Geometry check sheet. Reference: the model listing, model coordinates, mm. A direction names the side the tool comes from. Round coordinates to 2 decimals unless told otherwise and drop trailing zeros. Order: outer loops, then holes, each group sorted by start corner. A loop starts at its lowest first (then second) coordinate and runs counter-clockwise, first axis right, second up. Notation, with made-up numbers: (11.25, 31.25) -> (52.25, 31.25) arc R25 cw to (52.25, 52.25) -> close; hole circle Ø2 at (15, 60). An arc over 180 degrees is marked (long way). Use a Markdown table: item, result. Add a question column.
Item 1: Sectioned sample at B-B, the plane y = 22. Record the cut outline in (x, z).
Item 2: Sectioned sample at A-A, the plane x = 53. Record the cut outline in (y, z).
Item 3: Sectioned sample at C-C, the plane z = -48.5. Record the cut outline in (x, y).
Item 4: Material ranges on probe 1 along Z at (x, y) = (94, 0.8); probe 2 along Z at (x, y) = (68, 0.95); probe 3 along X at (y, z) = (0.85, 83), recorded low to high. Write a range as [from, to].
Item 5: Set-up check for faces 1 (the flat face through (63, 19, 74.035)), 2 (the flat face through (1, 0, 1)): record each of +Z, -Z, +X, -X, +Y, -Y from which the full face is reachable in a straight line by a thin tool's end or side.
Item 6: Gauge pin test, flat ends, axial feed: pin 1 Ø1.6 at (x, z) = (-94, -19.8) entering from -Y; pin 2 Ø2.5 at (x, z) = (98, -10) entering from -Y; pin 3 Ø4.5 at (y, z) = (16, 75.5) entering from -X; pin 4 Ø2.5 at (x, z) = (-94, -98.8) entering from +Y. Record the tip position at first contact, or that the pin passes through.
Autodesk Inventor part; units mm, degrees
ref_plane "YZ Plane" through (0, 0, 0) normal (1, 0, 0) x (0, 1, 0)
ref_plane "XZ Plane" through (0, 0, 0) normal (0, 1, 0) x (-1, 0, 0)
ref_plane "XY Plane" through (0, 0, 0) normal (0, 0, 1) x (1, 0, 0)
sketch "Sketch1" plane through (0, 0, 0) normal (0, 1, 0) x (-1, 0, 0)
  line L0 (100, -105) -> (-100, -105)
  line L1 (-100, -105) -> (-100, 105)
  line L2 (-100, 105) -> (100, 105)
  line L3 (100, 105) -> (100, -105)
  line L4 (100, -105) -> (-100, 105) construction
  line L5 (-100, -105) -> (100, 105) construction
  line L6 (-42.3092, 89.0348) -> (-82.3092, 89.0348)
  line L7 (-82.3092, 89.0348) -> (-82.3092, 74.0348)
  line L8 (-82.3092, 74.0348) -> (-42.3092, 74.0348)
  line L9 (-42.3092, 74.0348) -> (-42.3092, 89.0348)
  line L10 (-42.3092, 89.0348) -> (-82.3092, 74.0348) construction
  line L11 (-82.3092, 89.0348) -> (-42.3092, 74.0348) construction
  circle A0 centre (98, 83) radius 1
  circle A1 centre (98, 102.9) radius 1
  circle A2 centre (68, 102.9) radius 1
  circle A3 centre (-98, 102.9) radius 1
  circle A4 centre (-68, 102.9) radius 1
  circle A5 centre (98, -10) radius 1
  circle A6 centre (98, -55) radius 1
  circle A7 centre (-98, 83) radius 1
  circle A8 centre (-98, -10) radius 1
  circle A9 centre (-98, -55) radius 1
  circle A10 centre (-98, -102.9) radius 1.0002
  circle A11 centre (98, -102.9) radius 1
  circle A12 centre (-68, -102.9) radius 1
  circle A13 centre (0, -102.9) radius 1
  circle A14 centre (68, -102.9) radius 1
  line L12 (96, 61.2) -> (96, -100.8)
  circle A15 centre (94, -98.8) radius 1
  circle A16 centre (-94, -98.8) radius 1
  circle A17 centre (-94, 59.2) radius 1
  circle A18 centre (94, 59.2) radius 1
  circle A19 centre (94, -60.8) radius 1
  circle A20 centre (94, -19.8) radius 1
  circle A21 centre (94, 21.2) radius 1
  circle A22 centre (-94, -60.8) radius 1
  circle A23 centre (-94, -19.8) radius 1
  circle A24 centre (-94, 21.2) radius 1
  circle A25 centre (0, 59.2) radius 1
  circle A26 centre (0, -98.8) radius 1
  circle A27 centre (-48, 59.2) radius 1
  circle A28 centre (-48, -98.8) radius 1
  circle A29 centre (48, 59.2) radius 1
  circle A30 centre (48, -98.8) radius 1
  point P0 (0, 0)
  point P1 (-62.3092, 81.5348)
  dimension "d0" = 200
  dimension "d1" = 210
  dimension "d2" = 40
  dimension "d3" = 15
  dimension "d6" = 2
  dimension "d7" = 22
  dimension "d8" = 2
  dimension "d9" = 2
  dimension "d10" = 2.1
  dimension "d11" = 2
  dimension "d12" = 32
  dimension "d13" = 2.1
  dimension "d14" = 2
  dimension "d15" = 2.1
  dimension "d16" = 2
  dimension "d17" = 32
  dimension "d18" = 2.1
  dimension "d19" = 2
  dimension "d20" = 2
  dimension "d21" = 95
  dimension "d22" = 2
  dimension "d23" = 50
  dimension "d24" = 2
  dimension "d25" = 22
  dimension "d26" = 2
  dimension "d27" = 2
  dimension "d28" = 2
  dimension "d29" = 95
  dimension "d30" = 2
  dimension "d31" = 2
  dimension "d32" = 50
  dimension "d33" = 2
  dimension "d34" = 2.1
  dimension "d35" = 2.0005
  dimension "d36" = 2
  dimension "d38" = 2.1
  dimension "d39" = 2
  dimension "d40" = 32
  dimension "d41" = 2.1
  dimension "d42" = 2
  dimension "d43" = 2.1
  dimension "d44" = 100
  dimension "d45" = 2
  dimension "d46" = 2.1
  dimension "d47" = 32
  dimension "d56" = 2
  dimension "d59" = 6
  dimension "d60" = 6.2
  dimension "d61" = 2
  dimension "d64" = 6.2
  dimension "d65" = 6
  dimension "d66" = 2
  dimension "d69" = 6
  dimension "d70" = 45.8
  dimension "d71" = 2
  dimension "d74" = 6
  dimension "d75" = 45.8
  dimension "d77" = 2
  dimension "d79" = 2
  dimension "d80" = 2
  dimension "d84" = 2
  dimension "d87" = 2
  dimension "d90" = 2
  dimension "d93" = 2
extrude "MainBody" add sketch "Sketch1" along normal blind 3
sketch "Sketch2" plane through (0, 3, 0) normal (0, 1, 0) x (1, 0, 0)
  line L0 (82.3092, -74.0348) -> (82.3092, -89.0348)
  line L1 (82.3092, -74.0348) -> (42.3092, -74.0348)
  line L2 (42.3092, -74.0348) -> (42.3092, -78.0348)
  line L3 (42.3092, -78.0348) -> (82.3092, -78.0348)
  line L4 (82.3092, -78.0348) -> (82.3092, -74.0348)
  point P0 (0, 0)
  dimension "d48" = 4
  dimension "d49" = 40
extrude "Extrusion2" add sketch "Sketch2" along normal blind 32 and the other way blind 3
properties part number "DesignAtasRobot"
Found:
| question | item | result |
|---|---|---|
| 1 | outline | (42.31, 74.03) -> (82.31, 74.03) -> (82.31, 78.03) -> (42.31, 78.03) -> close |
| 2 | outline | (0, -105) -> (3, -105) -> (3, 74.03) -> (35, 74.03) -> (35, 78.03) -> (0, 78.03) -> close; (0, 89.03) -> (3, 89.03) -> (3, 105) -> (0, 105) -> close |
| 3 | outline | (-100, 0) -> (100, 0) -> (100, 3) -> (-100, 3) -> close |
| 4 | probe 1 | z = [-105, -99.8], [-97.8, -61.8], [-59.8, -20.8], [-18.8, 20.2], [22.2, 58.2], [60.2, 105] |
| 4 | probe 2 | z = [-105, -103.9], [-101.9, 78.03], [89.03, 101.9], [103.9, 105] |
| 4 | probe 3 | x = [-100, -99], [-97, 42.31], [82.31, 97], [99, 100] |
| 5 | face 1 | -Z, +X, -X, +Y |
| 5 | face 2 | +Z, -Z, +X, -X, -Y |
| 6 | pin 1 | passes through |
| 6 | pin 2 | stops at y = 0 |
| 6 | pin 3 | stops at x = 42.31 |
| 6 | pin 4 | stops at y = 3 |
